from build123d import *

# Parameters (mm, degrees)
SKETCH1_W                    = 45.72
SKETCH1_H                    = 120.65
BOSS_EXTRUDE1_DEPTH          = 3.175
SKETCH2_W                    = 45.72
SKETCH2_H                    = 3.175
BOSS_EXTRUDE2_DEPTH          = 7.62
SKETCH3_W                    = 10.795
SKETCH3_H                    = 15.875
CUT_EXTRUDE1_DEPTH           = 9.525
M4_CLEARANCE_HOLE1_D         = 4.5
FILLET1_R                    = 3.175
FILLET2_R                    = 3.175
M2_5X0_45_TAPPED_HOLE1_D     = 2.05
M2_5X0_45_TAPPED_HOLE1_DEPTH = 6.35
M2_5X0_45_TAPPED_HOLE1_TIP   = 0.615882135
SKETCH10_W                   = 33.02
SKETCH10_H                   = 40.005
CUT_EXTRUDE2_DEPTH           = 65.959599945
FILLET3_R                    = 6.35


with BuildPart() as part:
    # Sketch1 → Boss-Extrude1 (new body)
    with BuildSketch(Plane(origin=(0, 0, 0), x_dir=(0, 0, -1), z_dir=(1, 0, 0))):
        Rectangle(SKETCH1_W, SKETCH1_H)
    extrude(amount=BOSS_EXTRUDE1_DEPTH)

    # Sketch2 → Boss-Extrude2 (add)
    with BuildSketch(Plane(origin=(3.175, 0, 0), x_dir=(0, 0, -1), z_dir=(1, 0, 0))):
        with Locations((0, -58.7375)):
            Rectangle(SKETCH2_W, SKETCH2_H)
    extrude(amount=BOSS_EXTRUDE2_DEPTH)

    # Sketch3 → Cut-Extrude1 (cut)
    with BuildSketch(Plane.XZ.offset(60.325)):
        with Locations((5.3975, 0)):
            Rectangle(SKETCH3_W, SKETCH3_H)
    extrude(amount=-CUT_EXTRUDE1_DEPTH, mode=Mode.SUBTRACT)

    # M4 Clearance Hole1 (through all)
    with Locations(Plane(origin=(0, -57.15, 0), x_dir=(-1, 0, 0), z_dir=(0, 1, 0))):
        with Locations((-6.985, -13.7560191), (-6.985, 16.2960191)):
            Hole(M4_CLEARANCE_HOLE1_D / 2)

    # Fillet1
    fillet1_edges = [part.edges().sort_by_distance(p)[0] for p in [
        (1.5875, -50.8, -7.9375),
        (1.5875, -50.8, 7.9375),
    ]]
    fillet(fillet1_edges, radius=FILLET1_R)

    # Fillet2
    fillet2_edges = [part.edges().sort_by_distance(p)[0] for p in [
        (10.795, -58.7375, -22.86),
        (10.795, -58.7375, -7.9375),
        (10.795, -58.7375, 22.86),
        (10.795, -58.7375, 7.9375),
    ]]
    fillet(fillet2_edges, radius=FILLET2_R)

    # M2.5x0.45 Tapped Hole1
    with Locations(Plane(origin=(3.175, 0, 0), x_dir=(0, 0, -1), z_dir=(1, 0, 0))):
        with Locations((-13.585, -47.625), (18.415, -47.625), (18.415, -0.625), (-13.585, -0.625), (-13.585, 9.375), (18.415, 9.375), (18.415, 56.375), (-13.585, 56.375)):
            Hole(M2_5X0_45_TAPPED_HOLE1_D / 2, depth=M2_5X0_45_TAPPED_HOLE1_DEPTH)
            with Locations((0, 0, -(M2_5X0_45_TAPPED_HOLE1_DEPTH + M2_5X0_45_TAPPED_HOLE1_TIP / 2))):  # 118° drill point
                Cone(0, M2_5X0_45_TAPPED_HOLE1_D / 2, M2_5X0_45_TAPPED_HOLE1_TIP, mode=Mode.SUBTRACT)

    # Sketch10 → Cut-Extrude2 (cut, through all)
    with BuildSketch(Plane(origin=(3.175, 0, 0), x_dir=(0, 0, -1), z_dir=(1, 0, 0))):
        with Locations((0, 32.7025)):
            Rectangle(SKETCH10_W, SKETCH10_H)
        with Locations((0, -23.1775)):
            Rectangle(SKETCH10_W, SKETCH10_H)
    extrude(amount=-CUT_EXTRUDE2_DEPTH, mode=Mode.SUBTRACT)

    # Fillet3
    fillet3_edges = [part.edges().sort_by_distance(p)[0] for p in [
        (1.5875, 52.705, -16.51),
        (1.5875, 12.7, -16.51),
        (1.5875, 12.7, 16.51),
        (1.5875, 52.705, 16.51),
        (1.5875, -3.175, -16.51),
        (1.5875, -43.18, -16.51),
        (1.5875, -43.18, 16.51),
        (1.5875, -3.175, 16.51),
    ]]
    fillet(fillet3_edges, radius=FILLET3_R)


solid = part.part
Source: CAD feature listing. Evaluate the final solid. Frame: model axes, mm. A direction names the side the tool comes from. Round coordinates to 2 decimals unless told otherwise and drop trailing zeros. Loops run counter-clockwise (first coordinate to the right, second up) from the corner with the lowest first, then second, coordinate; pieces in that order, holes last. Notation, with made-up numbers: M 24.5,27 L 55.5,27 A12 ccw 55.5,36 Z; hole C -29.75,-10.5 d4. An arc over 180 degrees is marked long. Return JSON: item names as keys, results as strings. Group by question number.
1. Mould query, pull axis Z, two halves, no side actions, for faces 6 (the face through (5.199, -58.76, -15.125)), 7 (the face through (9.84, -58.715, 21.955)), 8 (the face through (10.795, -59, -15)), 9 (the face through (1.565, -46.761, 14.136)). Classes: released by +Z, released by -Z, zero draft, split by the parting line, or undercut.
2. Material intervals for line 1 along Z through (x, y) = (2.5, 26); line 2 along Y through (x, z) = (2, 16) (3 decimals); line 3 along Z through (x, y) = (3, -54.5), sorted ascending. Write a range as from..to.
3. Section query C-C on y = -42. Output: boundary loops of the cut face in (x, z) (3 decimals), and give its area (3 significant figures).
4. Pin query (flat end, axial travel): pin 1 (2 mm diameter, centred on y = -9.5, z = 16, fed in from +X) (3 decimals); pin 2 (3.5 mm diameter, centred on x = 1.5, z = 1, fed in from -Y). Return the tip coordinate at first contact, or that it passes through.
5. Section query B-B on z = 1. Output: boundary loops of the cut face in (x, y) (3 decimals).
6. Section query A-A on y = 30. Output: boundary loops of the cut face in (x, z) (3 decimals).
7. Reachability of faces 1 (the face through (9.84, -58.715, -21.955)), 2 (the face through (2, -50.8, 0)), 3 (the face through (2, 52.705, 0)), 4 (the face through (7, -57.15, -17)), 5 (the face through (9.84, -58.72, 8.84)) from +Z, -Z, +X, -X, +Y, -Y: full face, straight path, thin tool, end or side. Return the list, or none.
Checks:
{
 "1": {"face 6": "undercut", "face 7": "released by +Z", "face 8": "zero draft", "face 9": "undercut"},
 "2": {"line 1": "z = -22.86..-16.51, 16.51..22.86", "line 2": "y = -60.325..-39.323, -7.032..16.557, 48.848..60.325", "line 3": "z = -22.86..-7.94, 7.94..22.86"},
 "3": {"outline": "M 0,-22.86 L 3.175,-22.86 L 3.175,-13.847 L 0,-13.847 Z; M 0,13.847 L 3.175,13.847 L 3.175,22.86 L 0,22.86 Z", "area": "57.2 mm²"},
 "4": {"pin 1": "stops at x = 3.175", "pin 2": "stops at y = -50.8"},
 "5": {"outline": "M 0,-50.8 L 3.175,-50.8 L 3.175,-43.18 L 0,-43.18 Z; M 0,-3.175 L 3.175,-3.175 L 3.175,12.7 L 0,12.7 Z; M 0,52.705 L 3.175,52.705 L 3.175,60.325 L 0,60.325 Z"},
 "6": {"outline": "M 0,-22.86 L 3.175,-22.86 L 3.175,-16.51 L 0,-16.51 Z; M 0,16.51 L 3.175,16.51 L 3.175,22.86 L 0,22.86 Z"},
 "7": {"face 1": "-Z, +X, +Y, -Y", "face 2": "+X, -X, -Y", "face 3": "+X, -X", "face 4": "+Z, -Z, +X, +Y", "face 5": "+X, +Y, -Y"}
}
